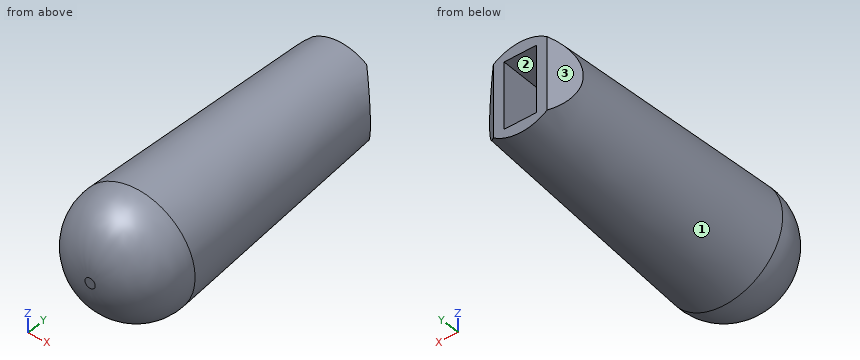
from build123d import *

# Parameters (mm, degrees)
SKETCH1_R           = 8.5
BOSS_EXTRUDE1_DEPTH = 57
BOSS_EXTRUDE1_TAPER = -3
FILLET1_R           = 10
CUT_EXTRUDE1_DEPTH  = 3
CUT_EXTRUDE2_DEPTH  = 23


with BuildPart() as part:
    # Sketch1 → Boss-Extrude1 (new body)
    with BuildSketch(Plane(origin=(0, 0, 0), x_dir=(1, 0, 0), z_dir=(0, 1, 0))):
        Circle(SKETCH1_R)
    extrude(amount=-BOSS_EXTRUDE1_DEPTH, taper=BOSS_EXTRUDE1_TAPER)

    # Fillet1
    fillet1_edges = [part.edges().sort_by_distance(p)[0] for p in [
        (-11.487243419, -57, 0),
    ]]
    fillet(fillet1_edges, radius=FILLET1_R)

    # Sketch2 → Cut-Extrude1 (cut, symmetric)
    with BuildSketch(Plane(origin=(0, 0, 0), x_dir=(0, 0, -1), z_dir=(1, 0, 0))):
        with BuildLine():
            Line((-6.3, 0), (6.3, 0))
            Line((6.3, 0), (6.3, -46.476640438))
            ThreePointArc((6.3, -46.476640438), (0, -52.776640438), (-6.3, -46.476640438))
            Line((-6.3, -46.476640438), (-6.3, 0))
        make_face()
    extrude(amount=CUT_EXTRUDE1_DEPTH, both=True, mode=Mode.SUBTRACT)

    # Sketch3 → Cut-Extrude2 (cut, symmetric)
    with BuildSketch(Plane.XY):
        Polygon((-5, 0), (5, 0), (10, -5), (10, 5), (-10, 5), (-10, -5), align=None)
    extrude(amount=CUT_EXTRUDE2_DEPTH, both=True, mode=Mode.SUBTRACT)


solid = part.part
Source: CAD feature listing. Evaluate the final solid. Frame: model axes, mm. Face numbers are marked on the shaded views. Round coordinates to 2 decimals unless told otherwise and drop trailing zeros. Loops run counter-clockwise (first coordinate to the right, second up) from the corner with the lowest first, then second, coordinate; pieces in that order, holes last. Notation, with made-up numbers: (25.25, 84) -> (63.25, 84) arc R10 ccw to (63.25, 89) -> close; hole circle Ø9 at (-28, -6.5). An arc over 180 degrees is marked (long way). Answer as a JSON object with one key per item and string values. Group by question number.
Q1. Section query B-B (y = -23). Output: boundary loops of the cut face in (x, z), plus the area to 3 significant figures.
Q2. Mould query, pull axis Z, two halves, no side actions, for the marked faces 1, 2 and 3. Classes: pulls with the +Z half, pulls with the -Z half, needs draft (parallel to the pull), parting line crosses it, or undercut.
Q3. Section query A-A (y = -32.5). Output: boundary loops of the cut face in (x, z), plus the area to 3 significant figures.
Q4. Contact query for flat-ended pins moving along their axis: P1, Ø6, axis at x = -6, z = 5.5, coming from the -Y side; P2, Ø5, axis at x = -2.5, y = -46, coming from the -Z side; P3, Ø5, axis at x = 5.5, y = -30.5, coming from the +Z side. Output: stop coordinate, or through.
Q5. Ray query, line 1 (Z direction, x = 0.75, y = -10); line 2 (X direction, y = -34.5, z = 1.25); line 3 (X direction, y = -13, z = 3.5). Return the intervals inside material, ascending. Write a range as from..to.
Completed:
{
 "1": {"outline": "circle Ø19.41 at (0, 0); hole (-3, -6.3) -> (3, -6.3) -> (3, 6.3) -> (-3, 6.3) -> close", "area": "220 mm²"},
 "2": {"face 1": "parting line crosses it", "face 2": "undercut", "face 3": "needs draft"},
 "3": {"outline": "circle Ø20.41 at (0, 0); hole (-3, -6.3) -> (3, -6.3) -> (3, 6.3) -> (-3, 6.3) -> close", "area": "251 mm²"},
 "4": {"P1": "y = -56.08", "P2": "z = -10.95", "P3": "z = 9.65"},
 "5": {"line 1": "-8.99..-6.3, 6.3..8.99", "line 2": "-10.23..-3, 3..10.23", "line 3": "-8.49..-3, 3..8.49"}
}
